The drawing under review shows one solid part. Ordinate dimensions are in mm from its lowest x, y, z. A direction names the side the tool comes from. Round coordinates to 2 decimals unless told otherwise and drop trailing zeros. Write each loop counter-clockwise with the first axis right and the second up, starting at its lowest first coordinate (ties: lowest second). Pieces come first, ordered by that corner, then holes. Notation, with made-up numbers: (-7, 57) - (2, 57) arc R19 cw to (2, 83) - close; hole circle Ø3 at (1.25, 19.5). An arc over 180 degrees is marked (long way). Answer in a Markdown table with one row per item. Add a question column.
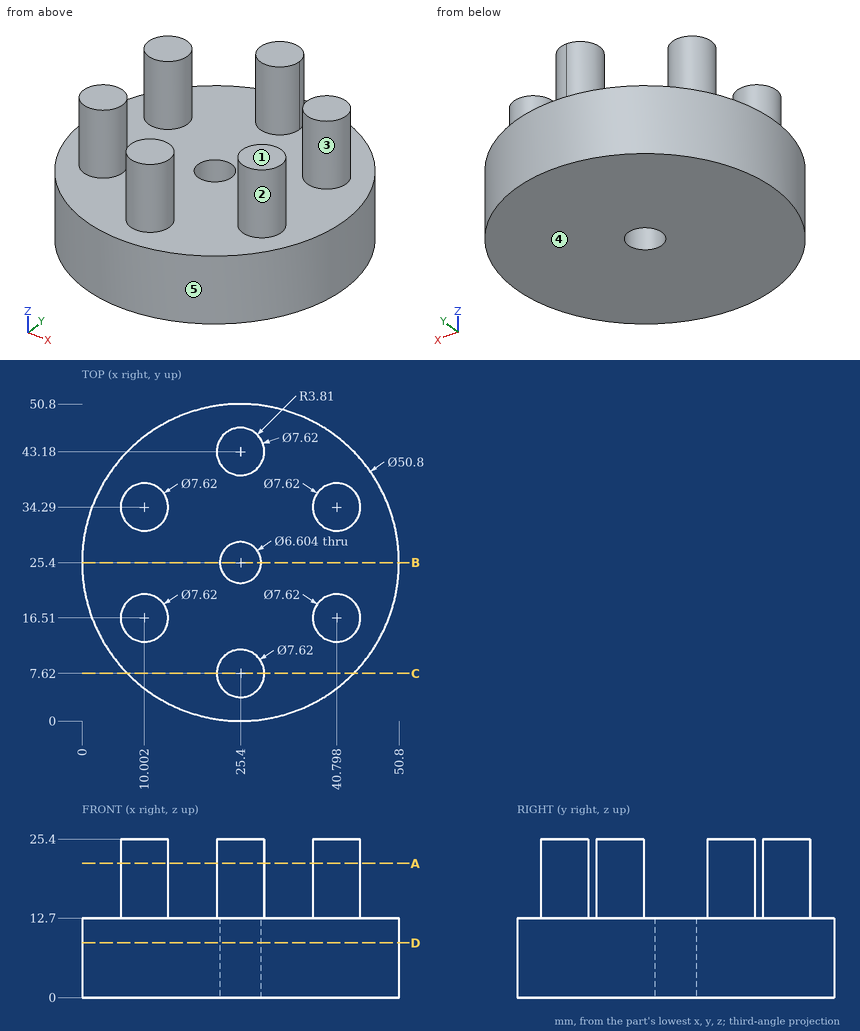
Q1. Add section D-D on z = 8.75. State the section outline as (x, y) points, then the cut area to 3 significant figures.
Q2. Tool access review of the marked faces 1 and 2: name each direction out of +Z, -Z, +X, -X, +Y, -Y from which nothing blocks a thin tool from reaching the whole face with its end or side.
Q3. To check wall thickness, follow probe 1 along Y at (x, z) = (25.4, 3.75); probe 2 along Z at (x, y) = (46.5, 24); probe 3 along X at (y, z) = (7.5, 23.75). State the ranges of each line that lie inside material, in increasing order.
Q4. Insertion check: pin 1 Ø12 at (x, y) = (16.5, 19) entering from -Z; pin 2 Ø4 at (y, z) = (38.5, 4.5) entering from +X; pin 3 Ø8 at (y, z) = (6.5, 12) entering from +X; pin 4 Ø2 at (x, z) = (18.5, 13) entering from +Y. Each pin has a flat end and moves straight along its axis. Give the tip position at first contact, or say it passes through.
Q5. Add section B-B on y = 25.4. State the section outline as (x, z) points.
Q6. Draft analysis for pull direction Y (two halves, no side actions). For the marked faces 3, 4 and 5, state which applies: released by +Y, released by -Y, zero draft, split by the parting line, or undercut.
Q7. Add section A-A on z = 21.5. State the section outline as (x, y) points.
Q8. Add section C-C on y = 7.62. State the section outline as (x, z) points, then the cut area to 4 significant figures.
Answer sheet:
| question | item | result |
|---|---|---|
| 1 | outline | circle Ø50.8 at (25.4, 25.4); hole circle Ø6.6 at (25.4, 25.4) |
| 1 | area | 1,990 mm² |
| 2 | face 1 | +Z, +X, -X, +Y, -Y |
| 2 | face 2 | +Z |
| 3 | probe 1 | y = 0 to 22.1, 28.7 to 50.8 |
| 3 | probe 2 | z = 0 to 12.7 |
| 3 | probe 3 | x = 21.59 to 29.21 |
| 4 | pin 1 | stops at z = 0 |
| 4 | pin 2 | stops at x = 48.25 |
| 4 | pin 3 | stops at x = 45.97 |
| 4 | pin 4 | stops at y = 50.09 |
| 5 | outline | (0, 0) - (22.1, 0) - (22.1, 12.7) - (0, 12.7) - close; (28.7, 0) - (50.8, 0) - (50.8, 12.7) - (28.7, 12.7) - close |
| 6 | face 3 | undercut |
| 6 | face 4 | zero draft |
| 6 | face 5 | split by the parting line |
| 7 | outline | circle Ø7.62 at (10, 16.51); circle Ø7.62 at (10, 34.29); circle Ø7.62 at (25.4, 7.62); circle Ø7.62 at (25.4, 43.18); circle Ø7.62 at (40.8, 16.51); circle Ø7.62 at (40.8, 34.29) |
| 8 | outline | (7.26, 0) - (43.54, 0) - (43.54, 12.7) - (29.21, 12.7) - (29.21, 25.4) - (21.59, 25.4) - (21.59, 12.7) - (7.26, 12.7) - close |
| 8 | area | 557.5 mm² |
